from build123d import *

# Parameters (mm, degrees)
SKETCH_1_W               = 48
SKETCH_1_H               = 45
EXTRUDE_1_DEPTH          = 10
SKETCH_2_R               = 2.5
CUT_EXTRUDE_1_DEPTH      = 1
CUT_EXTRUDE_1_DEPTH_BACK = 46
SKETCH_3_R               = 2
CUT_EXTRUDE_2_DEPTH      = 49
SKETCH_4_R               = 1.75
CUT_EXTRUDE_3_DEPTH      = 1.0000001
CUT_EXTRUDE_3_DEPTH_BACK = 49.0000001
SKETCH_5_W               = 17.7
SKETCH_5_H               = 17
CUT_EXTRUDE_4_DEPTH      = 11
SKETCH_6_W               = 17.7
SKETCH_6_H               = 1.5
SKETCH_6_H_2             = 2.5
CUT_EXTRUDE_5_DEPTH      = 11
SKETCH_8_R               = 2.5
EXTRUDE_2_DEPTH          = 45
SKETCH_10_R              = 1.75
CUT_EXTRUDE_8_DEPTH      = 45
SKETCH_16_W              = 38
SKETCH_16_H              = 37
CUT_EXTRUDE_13_DEPTH     = 11
SKETCH_17_W              = 38
SKETCH_17_H              = 10
SKETCH_17_R              = 1.75
EXTRUDE_4_DEPTH          = 3.5
SKETCH_18_W              = 38
SKETCH_18_H              = 10
SKETCH_18_R              = 1.75
EXTRUDE_5_DEPTH          = 2.5
FILLET_2_R               = 2
HOLE_WIZARD_M5_2_D       = 4.2
HOLE_WIZARD_M5_2_DEPTH   = 45
HOLE_WIZARD_M5_3_D       = 4.2
HOLE_WIZARD_M5_3_DEPTH   = 48
FILLET_3_R               = 2


with BuildPart() as part:
    # 草图1 → 凸台-拉伸1 (new body)
    with BuildSketch(Plane.XY):
        Rectangle(SKETCH_1_W, SKETCH_1_H)
    extrude(amount=EXTRUDE_1_DEPTH)

    # 草图2 → 切除-拉伸1 (cut, two sides)
    with BuildSketch(Plane(origin=(0, 22.5, 0), x_dir=(1, 0, 0), z_dir=(0, 1, 0))) as cut_extrude_1_sk:
        with Locations((10, -5)):
            Circle(SKETCH_2_R)
        with Locations((-10, -5)):
            Circle(SKETCH_2_R)
    extrude(amount=CUT_EXTRUDE_1_DEPTH, mode=Mode.SUBTRACT)
    extrude(cut_extrude_1_sk.sketch, amount=-CUT_EXTRUDE_1_DEPTH_BACK, mode=Mode.SUBTRACT)

    # 草图3 → 切除-拉伸2 (cut, through all)
    with BuildSketch(Plane(origin=(24, 0, 0), x_dir=(0, 0, -1), z_dir=(1, 0, 0))):
        with Locations((-5, -10.5)):
            Circle(SKETCH_3_R)
    extrude(amount=-CUT_EXTRUDE_2_DEPTH, mode=Mode.SUBTRACT)

    # 草图4 → 切除-拉伸3 (cut, two sides)
    with BuildSketch(Plane(origin=(24, 0, 0), x_dir=(0, 0, -1), z_dir=(1, 0, 0))) as cut_extrude_3_sk:
        with Locations((-5, 9.5)):
            Circle(SKETCH_4_R)
    extrude(amount=CUT_EXTRUDE_3_DEPTH, mode=Mode.SUBTRACT)
    extrude(cut_extrude_3_sk.sketch, amount=-CUT_EXTRUDE_3_DEPTH_BACK, mode=Mode.SUBTRACT)

    # 草图5 → 切除-拉伸4 (cut, through all)
    with BuildSketch(Plane.XY.offset(10)):
        with Locations((-10.15, -10.5)):
            Rectangle(SKETCH_5_W, SKETCH_5_H)
        with Locations((10.15, -10.5)):
            Rectangle(SKETCH_5_W, SKETCH_5_H)
        with Locations((-10.15, 9.5)):
            Rectangle(SKETCH_5_W, SKETCH_5_H)
        with Locations((10.15, 9.5)):
            Rectangle(SKETCH_5_W, SKETCH_5_H)
    extrude(amount=-CUT_EXTRUDE_4_DEPTH, mode=Mode.SUBTRACT)

    # 草图6 → 切除-拉伸5 (cut, through all)
    with BuildSketch(Plane.XY.offset(10)):
        with Locations((-10.15, 17.25)):
            Rectangle(SKETCH_6_W, SKETCH_6_H)
        with Locations((10.15, 17.25)):
            Rectangle(SKETCH_6_W, SKETCH_6_H)
        with Locations((-10.15, -0.25)):
            Rectangle(SKETCH_6_W, SKETCH_6_H_2)
        with Locations((10.15, -0.25)):
            Rectangle(SKETCH_6_W, SKETCH_6_H_2)
    extrude(amount=-CUT_EXTRUDE_5_DEPTH, mode=Mode.SUBTRACT)

    # 草图8 → 凸台-拉伸2 (add)
    with BuildSketch(Plane(origin=(0, 22.5, 0), x_dir=(1, 0, 0), z_dir=(0, 1, 0))):
        with Locations((10, -5)):
            Circle(SKETCH_8_R)
        with Locations((-10, -5)):
            Circle(SKETCH_8_R)
    extrude(amount=-EXTRUDE_2_DEPTH)

    # 草图10 → 切除-拉伸8 (cut)
    with BuildSketch(Plane(origin=(0, 22.5, 0), x_dir=(1, 0, 0), z_dir=(0, 1, 0))):
        with Locations((-7.5, -5)):
            Circle(SKETCH_10_R)
        with Locations((7.5, -5)):
            Circle(SKETCH_10_R)
    extrude(amount=-CUT_EXTRUDE_8_DEPTH, mode=Mode.SUBTRACT)

    # 草图16 → 切除-拉伸13 (cut, through all)
    with BuildSketch(Plane.XY.offset(10)):
        with Locations((0, -0.5)):
            Rectangle(SKETCH_16_W, SKETCH_16_H)
    extrude(amount=-CUT_EXTRUDE_13_DEPTH, mode=Mode.SUBTRACT)

    # 草图17 → 凸台-拉伸4 (add)
    with BuildSketch(Plane(origin=(0, -19, 0), x_dir=(1, 0, 0), z_dir=(0, 1, 0))):
        with Locations((0, -5)):
            Rectangle(SKETCH_17_W, SKETCH_17_H)
        with Locations((7.5, -5)):
            Circle(SKETCH_17_R, mode=Mode.SUBTRACT)
        with Locations((-7.5, -5)):
            Circle(SKETCH_17_R, mode=Mode.SUBTRACT)
    extrude(amount=EXTRUDE_4_DEPTH)

    # 草图18 → 凸台-拉伸5 (add)
    with BuildSketch(Plane.XZ.offset(-18)):
        with Locations((0, 5)):
            Rectangle(SKETCH_18_W, SKETCH_18_H)
        with Locations((-7.5, 5)):
            Circle(SKETCH_18_R, mode=Mode.SUBTRACT)
        with Locations((7.5, 5)):
            Circle(SKETCH_18_R, mode=Mode.SUBTRACT)
    extrude(amount=EXTRUDE_5_DEPTH)

    # 圆角2
    fillet_2_edges = [part.edges().sort_by_distance(p)[0] for p in [
        (-19, -15.5, 5),
        (19, -15.5, 5),
        (19, 15.5, 5),
        (-19, 15.5, 5),
    ]]
    fillet(fillet_2_edges, radius=FILLET_2_R)

    # M5 螺纹孔的螺纹孔钻头2
    with Locations(Plane(origin=(0, 22.5, 0), x_dir=(1, 0, 0), z_dir=(0, 1, 0))):
        with Locations((-7.5, -5), (7.5, -5)):
            Hole(HOLE_WIZARD_M5_2_D / 2, depth=HOLE_WIZARD_M5_2_DEPTH)

    # M5 螺纹孔的螺纹孔钻头3
    with Locations(Plane(origin=(24, 0, 0), x_dir=(0, 0, -1), z_dir=(1, 0, 0))):
        with Locations((-5, 9.5)):
            Hole(HOLE_WIZARD_M5_3_D / 2, depth=HOLE_WIZARD_M5_3_DEPTH)

    # 圆角3
    fillet_3_edges = [part.edges().sort_by_distance(p)[0] for p in [
        (24, -22.5, 5),
        (-24, -22.5, 5),
        (-24, 22.5, 5),
        (24, 22.5, 5),
    ]]
    fillet(fillet_3_edges, radius=FILLET_3_R)


solid = part.part
Model file for the job. Use its own axes, mm. A direction names the side the tool comes from. Give positions to 0.01 mm unless a question says otherwise; leave off trailing zeros. Write each loop counter-clockwise with the first axis right and the second up, starting at its lowest first coordinate (ties: lowest second). Pieces come first, ordered by that corner, then holes. Notation, with made-up numbers: (17.5, 86) -> (57.5, 86) arc R19 ccw to (57.5, 113) -> close; hole circle Ø3 at (-7, -12.75). An arc over 180 degrees is marked (long way). Write item = value, one per line.
(1) Slice it at D-D, the plane z = 1. Give the cut face in (x, y), then the cut area to 3 significant figures.
Determined:
outline = (-24, -20.5) arc R2 ccw to (-22, -22.5) -> (22, -22.5) arc R2 ccw to (24, -20.5) -> (24, 20.5) arc R2 ccw to (22, 22.5) -> (-22, 22.5) arc R2 ccw to (-24, 20.5) -> close; hole (-19, -13.5) arc R2 ccw to (-17, -15.5) -> (17, -15.5) arc R2 ccw to (19, -13.5) -> (19, 13.5) arc R2 ccw to (17, 15.5) -> (-17, 15.5) arc R2 ccw to (-19, 13.5) -> close
area = 982 mm2
(2) Slice it at C-C, the plane y = -7. Give the cut face in (x, z).
Determined:
outline = (-24, 0) -> (-19, 0) -> (-19, 10) -> (-24, 10) -> close; (19, 0) -> (24, 0) -> (24, 10) -> (19, 10) -> close
(3) Slice it at B-B, the plane x = -7.5. Give the cut face in (y, z).
Determined:
outline = (-22.5, 0) -> (-15.5, 0) -> (-15.5, 2.9) -> (-22.5, 2.9) -> close; (-22.5, 7.1) -> (-15.5, 7.1) -> (-15.5, 10) -> (-22.5, 10) -> close; (15.5, 0) -> (22.5, 0) -> (22.5, 2.9) -> (15.5, 2.9) -> close; (15.5, 7.1) -> (22.5, 7.1) -> (22.5, 10) -> (15.5, 10) -> close
(4) Probe line 1 along Y through (x, z) = (21.45, 5); line 2 along Y through (x, z) = (-6.5, 2.5); line 3 along Y through (x, z) = (22.95, 5). List the from-to ranges inside material, lowest first.
Determined:
line_1 = -22.5 to -12.5, -8.5 to 7.4, 11.6 to 22.5
line_2 = -22.5 to -15.5, 15.5 to 22.5
line_3 = -22.26 to -12.5, -8.5 to 7.4, 11.6 to 22.26
(5) Mould opens along X. For faces 1 (the face through (-21.465, -8.517, 5.26)), 2 (the face through (-5.834, 18.951, 6.278)), 3 (the face through (-24, 0, 5)), 4 (the face through (18.4, -14.93, 4.93)) say: released by +X, released by -X, zero draft, split by the parting line, or undercut.
Determined:
face_1 = zero draft
face_2 = undercut
face_3 = released by -X
face_4 = undercut
(6) Slice it at A-A, the plane y = 9.5. Give the cut face in (x, z).
Determined:
outline = (-24, 0) -> (-19, 0) -> (-19, 2.9) -> (-24, 2.9) -> close; (-24, 7.1) -> (-19, 7.1) -> (-19, 10) -> (-24, 10) -> close; (19, 0) -> (24, 0) -> (24, 2.9) -> (19, 2.9) -> close; (19, 7.1) -> (24, 7.1) -> (24, 10) -> (19, 10) -> close
(7) Tool access for faces 5 (the face through (23.43, -21.9, 5.07)), 6 (the face through (0, -15.5, 5)): list every direction of +Z, -Z, +X, -X, +Y, -Y with a clear straight run to the whole face (end or side of a thin tool).
Determined:
face_5 = +Z, -Z, +X, -Y
face_6 = +Z, -Z
